Model file for the job. Use its own axes, mm. A direction names the side the tool comes from. Coordinates: 2 decimals unless noted, no trailing zeros. Order: outer loops, then holes, each group sorted by start corner. A loop starts at its lowest first (then second) coordinate and runs counter-clockwise, first axis right, second up. Notation, with made-up numbers: (51, 57) -> (87, 57) arc R31 ccw to (87, 82) -> close; hole circle Ø1 at (35, -19.5). An arc over 180 degrees is marked (long way). Return JSON: item names as keys, results as strings. Group by question number.
1) Pull direction X, two halves, no side cores. Call faces 3 (the flat face through (0, 15, -37)), 4 (the flat face through (-4, 17, -37)), 5 (the flat face through (-76, 15, -38)): +X half, -X half, draft (parallel to the pull), parting line (faces both ways), or undercut.
2) Cut at C-C (y = 15). Write the cut outline in (x, z).
3) Cut at B-B (y = 5.25). Write the cut outline in (x, z), and give its area (3 significant figures).
4) Cut at A-A (x = -38). Write the cut outline in (y, z).
5) Which spindle directions (+Z, -Z, +X, -X, +Y, -Y) get a long thin tool onto all of the face, cutting with end or side? Do faces 1 (the flat face through (-29, 15, -75.928)), 2 (the flat face through (-38, 23, -3.928)). Say none if no direction does.
6) Flat gauge pin, fed straight in: pin 1 (20.5 mm diameter, centred on x = -51, z = -44, fed in from +Y). Where does the tip first touch, or does it go through?
7) Probe line 1 (X direction, y = 17.5, z = -53); line 2 (X direction, y = 15, z = -1.3); line 3 (Y direction, x = -38, z = -73.2). List the from-to ranges inside material, lowest first.
8) Cut at D-D (x = -11). Write the cut outline in (y, z).
Autodesk Inventor part; units mm, degrees
ref_plane "YZ Plane" through (0, 0, 0) normal (1, 0, 0) x (0, 1, 0)
ref_plane "XZ Plane" through (0, 0, 0) normal (0, 1, 0) x (-1, 0, 0)
ref_plane "XY Plane" through (0, 0, 0) normal (0, 0, 1) x (1, 0, 0)
sketch "Sketch1" plane through (0, 0, 0) normal (0, 1, 0) x (-1, 0, 0)
  line L0 (76, 0.0718) -> (0, 0.0718)
  line L1 (0, 0.0718) -> (0, -75.9282)
  line L2 (0, -75.9282) -> (76, -75.9282)
  line L3 (76, -75.9282) -> (76, 0.0718)
  point P0 (0, 0)
  dimension "d0" = 76
  dimension "d1" = 76
extrude "Extrusion1" add sketch "Sketch1" along normal blind 30
shell "Shell1" thickness 4 removed faces 1 at (-50.6667, 30, -25.2616)
sketch "Sketch2" plane through (-76, 0, 0.0718) normal (0, 0, 1) x (1, 0, 0)
  line L0 (0, 30) -> (76, 30)
  line L1 (38, 30) -> (38, 0)
  line L2 (0, 0) -> (76, 0)
  line L3 (0, 0) -> (0, 30)
  line L4 (0, 15) -> (76, 15)
  line L5 (76, 0) -> (76, 30)
  circle A0 centre (38, 15) radius 7.5
  dimension "d5" = 15
hole "Hole1" at (-38, 15, 0.0718) direction (0, 0, -1) diameter 15 end through all
properties part number "Caja_ampli_antena"
Answers below:
{
 "1": {"face 3": "+X half", "face 4": "undercut", "face 5": "-X half"},
 "2": {"outline": "(-76, -75.93) -> (-45.5, -75.93) -> (-45.5, -71.93) -> (-72, -71.93) -> (-72, -3.93) -> (-45.5, -3.93) -> (-45.5, 0.07) -> (-76, 0.07) -> close; (-30.5, -75.93) -> (0, -75.93) -> (0, 0.07) -> (-30.5, 0.07) -> (-30.5, -3.93) -> (-4, -3.93) -> (-4, -71.93) -> (-30.5, -71.93) -> close"},
 "3": {"outline": "(-76, -75.93) -> (0, -75.93) -> (0, 0.07) -> (-76, 0.07) -> close; hole (-72, -71.93) -> (-4, -71.93) -> (-4, -3.93) -> (-72, -3.93) -> close", "area": "1,150 mm^2"},
 "4": {"outline": "(0, -75.93) -> (7.5, -75.93) -> (7.5, -71.93) -> (4, -71.93) -> (4, -3.93) -> (7.5, -3.93) -> (7.5, 0.07) -> (0, 0.07) -> close; (22.5, -75.93) -> (30, -75.93) -> (30, -71.93) -> (22.5, -71.93) -> close; (22.5, -3.93) -> (30, -3.93) -> (30, 0.07) -> (22.5, 0.07) -> close"},
 "5": {"face 1": "-Z, +X, -X, +Y, -Y", "face 2": "+Y"},
 "6": {"pin 1": "stops at y = 4"},
 "7": {"line 1": "x = -76 to -72, -4 to 0", "line 2": "x = -76 to -45.5, -30.5 to 0", "line 3": "y = 0 to 7.5, 22.5 to 30"},
 "8": {"outline": "(0, -75.93) -> (30, -75.93) -> (30, -71.93) -> (4, -71.93) -> (4, -3.93) -> (30, -3.93) -> (30, 0.07) -> (0, 0.07) -> close"}
}
